```python
from build123d import *

# Parameters (mm, degrees)
F0_W      = 137.5
F0_H      = 84
F0_R      = 35.5
F1_DEPTH  = 2
F2_R      = 37.5
F4_R      = 23
F6_R      = 35.5
F7_R      = 21
F9_R      = 23
F9_R_2    = 12.864396
F10_DEPTH = 2


with BuildPart() as f1:
    # F0 (on Front) → F1 (new body)
    with BuildSketch(Plane.XZ):
        Rectangle(F0_W, F0_H)
        Circle(F0_R, mode=Mode.SUBTRACT)
    extrude(amount=F1_DEPTH)

    # F2 (on face) → F5 section 0
    with BuildSketch(Plane.XZ.offset(2)):
        Circle(F2_R)
    # F4 (on offset) → F5 section 1
    with BuildSketch(Plane.XZ.offset(42)):
        Circle(F4_R)
    loft()

    # F6 (on face) → F8 section 0
    with BuildSketch(Plane.XZ.offset(2)):
        Circle(F6_R)
    # F7 (on face) → F8 section 1
    with BuildSketch(Plane.XZ.offset(42)):
        Circle(F7_R)
    loft(mode=Mode.SUBTRACT)

    # F9 (on offset) → F10 (join)
    with BuildSketch(Plane.XZ.offset(42)):
        Circle(F9_R)
        Circle(F9_R_2, mode=Mode.SUBTRACT)
    extrude(amount=F10_DEPTH)


solid = f1.part
```
For this review, take the finished solid that the model builds, in its own axes (mm). A direction names the side the tool comes from. Round coordinates to 2 decimals unless told otherwise and drop trailing zeros. Order: outer loops, then holes, each group sorted by start corner. A loop starts at its lowest first (then second) coordinate and runs counter-clockwise, first axis right, second up. Notation, with made-up numbers: (88.25, 50.5) -> (98.25, 50.5) arc R26 ccw to (98.25, 66.5) -> close; hole circle Ø4 at (32, 13). An arc over 180 degrees is marked (long way). Use a Markdown table: item, result.
Item 1: Take a section at D-D (y = -24.5). State the section outline as (x, z) points, plus the area to 3 significant figures.
Resolved:
| item | result |
|---|---|
| outline | circle Ø58.69 at (0, 0); hole circle Ø54.69 at (0, 0) |
| area | 356 mm² |
Item 2: Take a section at B-B (y = -32). State the section outline as (x, z) points (3 decimals), plus the area to 3 significant figures.
Resolved:
| item | result |
|---|---|
| outline | circle Ø53.25 at (0, 0); hole circle Ø49.25 at (0, 0) |
| area | 322 mm² |
Item 3: Take a section at C-C (x = -51). State the section outline as (y, z) points.
Resolved:
| item | result |
|---|---|
| outline | (-2, -42) -> (0, -42) -> (0, 42) -> (-2, 42) -> close |
Item 4: For line 1 along Z through (x, y) = (0, -1.45); line 2 along Y through (x, z) = (23, -36); line 3 along Y through (x, z) = (-11.5, -7), list the stretches that pass through material, from the lowest coordinate up. Write a range as [from, to].
Resolved:
| item | result |
|---|---|
| line 1 | z = [-42, -35.5], [35.5, 42] |
| line 2 | y = [-2, 0] |
| line 3 | y = [-44, -42] |
Item 5: Machinability: for faces 4 (the cylindrical face through (-2.79, -42.99, -12.56)), 5 (the cylindrical face through (-7.696, -0.986, -34.656)), which of the approach directions +Z, -Z, +X, -X, +Y, -Y give a long, thin tool a straight path to every point of the face, cutting with its end or side? Answer none if there is none.
Resolved:
| item | result |
|---|---|
| face 4 | +Y, -Y |
| face 5 | +Y |
Item 6: For pin 1 (10 mm diameter, centred on x = -20, y = -39.5, fed in from -Z); pin 2 (5 mm diameter, centred on x = -13, y = -31, fed in from +Z); pin 3 (5 mm diameter, centred on y = -32, z = 10.5, fed in from +X), all flat-tipped, find the tip position at first contact; note any pin that passes through.
Resolved:
| item | result |
|---|---|
| pin 1 | stops at z = -19.24 |
| pin 2 | stops at z = 25.24 |
| pin 3 | stops at x = 25.83 |
Item 7: Take a section at A-A (x = 0). State the section outline as (y, z) points.
Resolved:
| item | result |
|---|---|
| outline | (-44, -23) -> (-42, -23) -> (-2, -37.5) -> (-2, -42) -> (0, -42) -> (0, -35.5) -> (-2, -35.5) -> (-42, -21) -> (-42, -12.86) -> (-44, -12.86) -> close; (-44, 12.86) -> (-42, 12.86) -> (-42, 21) -> (-2, 35.5) -> (0, 35.5) -> (0, 42) -> (-2, 42) -> (-2, 37.5) -> (-42, 23) -> (-44, 23) -> close |
Item 8: Draft analysis for pull direction X (two halves, no side actions). For faces 1 (the flat face through (9, -42, 10)), 2 (the cylindrical face through (-2.994, -42.986, 22.804)), 3 (the flat face through (-1, -2, 38)), state which applies: +X half, -X half, draft (parallel to the pull), parting line (faces both ways), or undercut.
Resolved:
| item | result |
|---|---|
| face 1 | undercut |
| face 2 | parting line |
| face 3 | draft |
